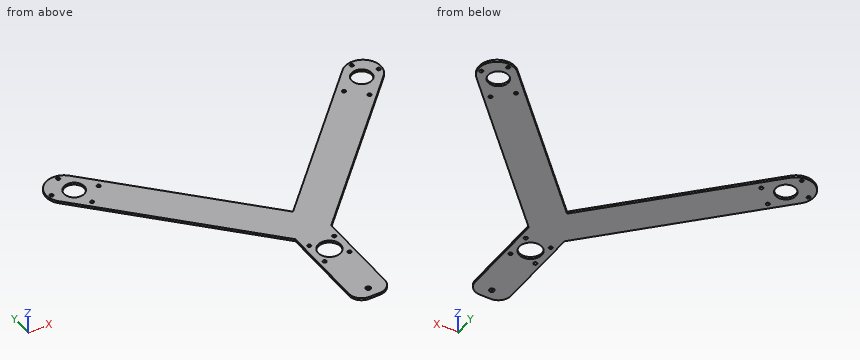
```python
from build123d import *

# Parameters (mm, degrees)
BOSS_EXTRUDE1_DEPTH = 3.175
SKETCH2_R           = 14.2875
SKETCH2_R_2         = 15.875
SKETCH2_R_3         = 2.54
CUT_EXTRUDE1_DEPTH  = 491.500657373
FILLET1_R           = 25.4
SKETCH7_R           = 3.556
CUT_EXTRUDE6_DEPTH  = 476.917284882
FILLET2_R           = 17.78
FILLET3_R           = 17.78
SKETCH9_R           = 2.54
CUT_EXTRUDE7_DEPTH  = 476.917284882


with BuildPart() as part:
    # Sketch1 → Boss-Extrude1 (new body)
    with BuildSketch(Plane.XY):
        Polygon((0, 0), (50.8, 0), (50.8, 141.300925348), (273.474793589, 371.887424227), (236.932331732, 407.176069446), (25.4, 188.127927591), (-186.132331732, 407.176069446), (-222.674793589, 371.887424227), (0, 141.300925348), align=None)
    extrude(amount=BOSS_EXTRUDE1_DEPTH)

    # Sketch2 → Cut-Extrude1 (cut, through all)
    with BuildSketch(Plane.XY.offset(3.175)):
        with Locations((232.265943268, 365.779146629)):
            Circle(SKETCH2_R)
        with Locations((-177.937078746, 362.124900444)):
            Circle(SKETCH2_R)
        with Locations((25.4, 104.14)):
            Circle(SKETCH2_R_2)
        with Locations((43.1292, 121.8692)):
            Circle(SKETCH2_R_3)
        with Locations((7.6708, 121.8692)):
            Circle(SKETCH2_R_3)
        with Locations((7.6708, 86.4108)):
            Circle(SKETCH2_R_3)
        with Locations((43.1292, 86.4108)):
            Circle(SKETCH2_R_3)
    extrude(amount=-CUT_EXTRUDE1_DEPTH, mode=Mode.SUBTRACT)

    # Fillet1
    fillet1_edges = [part.edges().sort_by_distance(p)[0] for p in [
        (273.474793589, 371.887424227, 1.5875),
        (236.932331732, 407.176069446, 1.5875),
        (-222.674793589, 371.887424227, 1.5875),
        (-186.132331732, 407.176069446, 1.5875),
    ]]
    fillet(fillet1_edges, radius=FILLET1_R - 0.0001)  # a hair under: the kernel refuses the full size

    # Sketch7 → Cut-Extrude6 (cut, through all)
    with BuildSketch(Plane(origin=(0, 0, 0), x_dir=(-1, 0, 0), z_dir=(0, 0, -1))):
        with Locations((-25.507732434, 14.949579081)):
            Circle(SKETCH7_R)
    extrude(amount=-CUT_EXTRUDE6_DEPTH, mode=Mode.SUBTRACT)

    # Fillet2
    fillet2_edges = [part.edges().sort_by_distance(p)[0] for p in [
        (0, 0, 1.5875),
    ]]
    fillet(fillet2_edges, radius=FILLET2_R)

    # Fillet3
    fillet3_edges = [part.edges().sort_by_distance(p)[0] for p in [
        (50.8, 0, 1.5875),
    ]]
    fillet(fillet3_edges, radius=FILLET3_R)

    # Sketch9 → Cut-Extrude7 (cut, through all)
    with BuildSketch(Plane(origin=(0, 0, 0), x_dir=(-1, 0, 0), z_dir=(0, 0, -1))):
        with Locations((-233.698211642, 390.878637547)):
            Circle(SKETCH9_R)
        with Locations((-257.542931638, 367.852059109)):
            Circle(SKETCH9_R)
        with Locations((-199.415247758, 353.365000514)):
            Circle(SKETCH9_R)
        with Locations((-222.254286418, 331.309597252)):
            Circle(SKETCH9_R)
    cut_extrude7 = extrude(amount=-CUT_EXTRUDE7_DEPTH, mode=Mode.SUBTRACT)

    # Mirror3: Cut-Extrude7 across plane
    add(cut_extrude7.mirror(Plane.ZY.offset(-25.4)), mode=Mode.SUBTRACT)


solid = part.part
```
Verification items for the finished model (mm, model axes). Round coordinates to 2 decimals unless told otherwise and drop trailing zeros. Write each loop counter-clockwise with the first axis right and the second up, starting at its lowest first coordinate (ties: lowest second). Pieces come first, ordered by that corner, then holes. Notation, with made-up numbers: (-3.5, -21.5) - (36.5, -21.5) arc R20 cw to (36.5, 8.5) - close; hole circle Ø3 at (76.5, 21). An arc over 180 degrees is marked (long way). Answer as a JSON object with one key per item and string values. Group by question number.
Q1. Section check C-C, the plane y = 55.5. Enter the section's corners in (x, z) (3 decimals), plus the area to 3 significant figures.
Q2. Thickness scan on line 1 (X direction, y = 87, z = 0.7); line 2 (X direction, y = 333, z = 2.55); line 3 (Y direction, x = 42.5, z = 1.8). Record the ranges inside material, lowest first.
Q3. Go/stop test with flat-tipped pins: pin 1 Ø3 at (x, y) = (53, 77) entering from -Z; pin 2 Ø1 at (x, z) = (-164.5, 2) entering from +Y; pin 3 Ø1.5 at (y, z) = (316, 1.5) entering from +X; pin 4 Ø6 at (x, y) = (257.54, 367.85) entering from -Z. Record where each tip stops, or that it passes through.
Q4. Section check B-B, the plane z = 2.5. Give the number of separate pieces and of enclosed holes in the cut face, plus the area to 3 significant figures.
Q5. Section check D-D, the plane x = -28. Enter the section's corners in (y, z) (3 decimals), plus the area to 3 significant figures.
Q6. Section check A-A, the plane y = 104.14. Enter the section's corners in (x, z) (3 decimals), plus the area to 3 significant figures.
Found:
{
 "1": {"outline": "(0, 0) - (50.8, 0) - (50.8, 3.175) - (0, 3.175) - close", "area": "161 mm^2"},
 "2": {"line 1": "x = 0 to 5.2, 10.14 to 40.66, 45.6 to 50.8", "line 2": "x = -185.12 to -173.35, -169.56 to -114.5, 165.3 to 220.36, 224.15 to 235.92", "line 3": "y = 2.74 to 83.95, 88.87 to 119.41, 124.33 to 205.84"},
 "3": {"pin 1": "passes through", "pin 2": "stops at y = 385.29", "pin 3": "stops at x = 220.23", "pin 4": "stops at z = 0"},
 "4": {"separate pieces": "1", "enclosed holes": "16", "area": "37,100 mm^2"},
 "5": {"outline": "(170.296, 0) - (243.425, 0) - (243.425, 3.175) - (170.296, 3.175) - close", "area": "232 mm^2"},
 "6": {"outline": "(0, 0) - (9.525, 0) - (9.525, 3.175) - (0, 3.175) - close; (41.275, 0) - (50.8, 0) - (50.8, 3.175) - (41.275, 3.175) - close", "area": "60.5 mm^2"}
}
